Read the model definition and answer for the solid it produces. Units are mm, in the model's axes. A direction names the side the tool comes from. Coordinates: 2 decimals unless noted, no trailing zeros. Order: outer loops, then holes, each group sorted by start corner. A loop starts at its lowest first (then second) coordinate and runs counter-clockwise, first axis right, second up. Notation, with made-up numbers: (61.25, 21.25) -> (93.25, 21.25) arc R26 ccw to (93.25, 54.25) -> close; hole circle Ø6 at (-8.5, -35.75). An arc over 180 degrees is marked (long way). Answer as a JSON object with one key per item and string values. Group by question number.
1) Section C-C on y = -10 is taken. Determine the outline of the cut face in (x, z).
2) Section B-B on z = -11.5 is taken. Determine the outline of the cut face in (x, y).
3) Determine the mould class of faces 5 (the flat face through (0, -30, 19.05)), 6 (the flat face through (20, -16.669, 8)), 7 (the cylindrical face through (20.09, -8.38, -14.41)), 8 (the flat face through (0, -33.782, 0)) for opening direction Y: released by +Y, released by -Y, zero draft, split by the parting line, or undercut.
4) Consider L1, parallel to Y at x = -13, z = -23.5; L2, parallel to X at y = -12.5, z = -26; L3, parallel to Y at x = 16, z = -26.5. Determine where each line is inside the solid, lowest interval first.
5) Section A-A on x = -6 is taken. Determine the outline of the cut face in (y, z) (3 decimals).
6) Given pin 1 (8 mm diameter, centred on x = 14.5, y = 4.5, fed in from -Z); pin 2 (10 mm diameter, centred on y = -7.5, z = -25.5, fed in from -X); pin 3 (4 mm diameter, centred on x = 15.5, z = -21.5, fed in from +Y); pin 4 (15.5 mm diameter, centred on x = -19.5, z = 9.5, fed in from +Y), each flat-ended and moving along its own axis, determine where each tip first touches the part or whether it passes through.
7) A tool of negligible diameter and unlimited length cuts with its end or side. For faces 1 (the cylindrical face through (-19.89, -17.49, 17.313)), 2 (the flat face through (26.988, -13, -13)), 3 (the cylindrical face through (18.297, -7.195, -22.343)), 4 (the cylindrical face through (-18.297, -7.195, -22.343)), from which of +Z, -Z, +X, -X, +Y, -Y can it reach the whole face along a straight path? Write none if from no direction.
from build123d import *

# Parameters (mm, degrees)
BOSS_EXTRUDE1_DEPTH = 26.9875
SKETCH2_R           = 3.175
BOSS_EXTRUDE2_DEPTH = 26.9875
CUT_EXTRUDE1_DEPTH  = 14
CUT_EXTRUDE2_START  = -39.975
CUT_EXTRUDE2_DEPTH  = 14
CUT_EXTRUDE3_DEPTH  = 17.6276
CUT_EXTRUDE4_START  = -53.975
CUT_EXTRUDE4_DEPTH  = 17.6276


with BuildPart() as part:
    # Sketch1 → Boss-Extrude1 (new, symmetric)
    with BuildSketch(Plane(origin=(0, 0, 0), x_dir=(0, 0, -1), z_dir=(1, 0, 0))):
        with BuildLine():
            Line((-15.761022628, 1.898891971), (-19.05, -25.4))
            Line((-19.05, -25.4), (-19.05, -33.782))
            Line((-19.05, -33.782), (19.05, -33.782))
            Line((19.05, -33.782), (19.05, -25.4))
            Line((19.05, -25.4), (15.761022628, 1.898891971))
            ThreePointArc((15.761022628, 1.898891971), (0, 15.875), (-15.761022628, 1.898891971))
        make_face()
    extrude(amount=BOSS_EXTRUDE1_DEPTH, both=True)

    # Sketch2 → Boss-Extrude2 (add, symmetric)
    with BuildSketch(Plane(origin=(0, 0, 0), x_dir=(0, 0, -1), z_dir=(1, 0, 0))):
        with BuildLine():
            Line((34.849752976, -7.546656143), (31.331707433, 16.706942484))
            ThreePointArc((31.331707433, 16.706942484), (29.318806596, 19.218576271), (26.145386515, 18.680543695))
            Line((26.145386515, 18.680543695), (13.625741227, 8.145845629))
            ThreePointArc((13.625741227, 8.145845629), (15.021703631, 5.134592976), (15.761022628, 1.898891971))
            Line((15.761022628, 1.898891971), (19.05, -25.4))
            Line((19.05, -25.4), (19.05, -33.782))
            Line((19.05, -33.782), (33.819378976, -12.024635583))
            ThreePointArc((33.819378976, -12.024635583), (34.753812672, -9.882113678), (34.849752976, -7.546656143))
        make_face()
        with Locations((28.565519705, -8.4582)):
            Circle(SKETCH2_R, mode=Mode.SUBTRACT)
    extrude(amount=BOSS_EXTRUDE2_DEPTH, both=True)

    # Sketch3 → Cut-Extrude1 (cut)
    with BuildSketch(Plane(origin=(26.9875, 0, 0), x_dir=(0, 0, -1), z_dir=(1, 0, 0))):
        with BuildLine():
            Line((-15.18262128, -16.66875), (0, -16.66875))
            ThreePointArc((0, -16.66875), (14.530186835, -8.168286057), (14.240626625, 8.663243036))
            Line((14.240626625, 8.663243036), (13.625741227, 8.145845629))
            ThreePointArc((13.625741227, 8.145845629), (-3.300903538, 15.528028234), (-15.761022628, 1.898891971))
            Line((-15.761022628, 1.898891971), (-18.334825806, -19.463971606))
            ThreePointArc((-18.334825806, -19.463971606), (-17.289138382, -17.468205704), (-15.18262128, -16.66875))
        make_face()
    extrude(amount=-CUT_EXTRUDE1_DEPTH, mode=Mode.SUBTRACT)

    # Sketch3<3> → Cut-Extrude2 (cut)
    with BuildSketch(Plane(origin=(26.9875, 0, 0), x_dir=(0, 0, -1), z_dir=(1, 0, 0)).offset(CUT_EXTRUDE2_START)):
        with BuildLine():
            Line((-15.18262128, -16.66875), (0, -16.66875))
            ThreePointArc((0, -16.66875), (14.530186835, -8.168286057), (14.240626625, 8.663243036))
            Line((14.240626625, 8.663243036), (13.625741227, 8.145845629))
            ThreePointArc((13.625741227, 8.145845629), (-3.300903538, 15.528028234), (-15.761022628, 1.898891971))
            Line((-15.761022628, 1.898891971), (-18.334825806, -19.463971606))
            ThreePointArc((-18.334825806, -19.463971606), (-17.289138382, -17.468205704), (-15.18262128, -16.66875))
        make_face()
    extrude(amount=-CUT_EXTRUDE2_DEPTH, mode=Mode.SUBTRACT)

    # Sketch4 → Cut-Extrude3 (cut)
    with BuildSketch(Plane(origin=(26.9875, 0, 0), x_dir=(0, 0, -1), z_dir=(1, 0, 0))):
        with BuildLine():
            Line((33.819378976, -12.024635583), (30.252943393, -17.278494853))
            ThreePointArc((30.252943393, -17.278494853), (30.324357139, -15.61082693), (28.864686801, -14.801148766))
            ThreePointArc((28.864686801, -14.801148766), (22.377226739, -7.034286322), (31.606824582, -2.883887069))
            ThreePointArc((31.606824582, -2.883887069), (33.273576843, -2.793592413), (33.938209118, -1.262422872))
            Line((33.938209118, -1.262422872), (34.849752976, -7.546656143))
            ThreePointArc((34.849752976, -7.546656143), (34.753812672, -9.882113678), (33.819378976, -12.024635583))
        make_face()
    extrude(amount=-CUT_EXTRUDE3_DEPTH, mode=Mode.SUBTRACT)

    # Sketch5<3> → Cut-Extrude4 (cut)
    with BuildSketch(Plane(origin=(26.9875, 0, 0), x_dir=(0, 0, -1), z_dir=(1, 0, 0)).offset(CUT_EXTRUDE4_START)):
        with BuildLine():
            Line((33.819378976, -12.024635583), (30.252943393, -17.278494853))
            ThreePointArc((30.252943393, -17.278494853), (30.324357139, -15.61082693), (28.864686801, -14.801148766))
            ThreePointArc((28.864686801, -14.801148766), (22.377226739, -7.034286322), (31.606824582, -2.883887069))
            ThreePointArc((31.606824582, -2.883887069), (33.273576843, -2.793592413), (33.938209118, -1.262422872))
            Line((33.938209118, -1.262422872), (34.849752976, -7.546656143))
            ThreePointArc((34.849752976, -7.546656143), (34.753812672, -9.882113678), (33.819378976, -12.024635583))
        make_face()
    extrude(amount=CUT_EXTRUDE4_DEPTH, mode=Mode.SUBTRACT)


solid = part.part
Worked answers:
{
 "1": {"outline": "(-26.99, -22.41) -> (-9.36, -22.41) -> (-9.36, -25.79) -> (9.36, -25.79) -> (9.36, -22.41) -> (26.99, -22.41) -> (26.99, -13.34) -> (12.99, -13.34) -> (12.99, 17.19) -> (-12.99, 17.19) -> (-12.99, -13.34) -> (-26.99, -13.34) -> close; (-9.36, -34.73) -> (9.36, -34.73) -> (9.36, -31.34) -> (-9.36, -31.34) -> close"},
 "2": {"outline": "(-26.99, -33.78) -> (26.99, -33.78) -> (26.99, -12.07) -> (12.99, -12.07) -> (12.99, 10.94) -> (-12.99, 10.94) -> (-12.99, -12.07) -> (-26.99, -12.07) -> close"},
 "3": {"face 5": "zero draft", "face 6": "released by +Y", "face 7": "undercut", "face 8": "released by -Y"},
 "4": {"L1": "y = -27.23 to -12.29, -4.63 to 16.45", "L2": "x = -9.36 to 9.36", "L3": "y = -22.81 to -14.46, -2.45 to 18.94"},
 "5": {"outline": "(-33.782, -19.05) -> (-12.025, -33.819) arc R6.35 ccw to (-7.547, -34.85) -> (16.707, -31.332) arc R3.175 ccw to (18.681, -26.145) -> (8.146, -13.626) arc R15.875 ccw to (1.899, 15.761) -> (-25.4, 19.05) -> (-33.782, 19.05) -> close; hole circle Ø6.35 at (-8.458, -28.566)"},
 "6": {"pin 1": "stops at z = -33.68", "pin 2": "stops at x = -26.99", "pin 3": "stops at y = 16.45", "pin 4": "stops at y = 14.96"},
 "7": {"face 1": "+Z, -X, +Y", "face 2": "+Z, -Z, +X, +Y, -Y", "face 3": "+X", "face 4": "-X"}
}
